Here's how the part is built. I have some questions about the finished solid (model axes, mm). A direction names the side the tool comes from. Round coordinates to 2 decimals unless told otherwise and drop trailing zeros. Loops run counter-clockwise (first coordinate to the right, second up) from the corner with the lowest first, then second, coordinate; pieces in that order, holes last. Notation, with made-up numbers: M -28.75,-11.5 L 30.25,-11.5 A15 cw 30.25,5.5 Z; hole C 72.25,42.25 d1. An arc over 180 degrees is marked long. Write each question's results on one line, items separated by ' | '. Start each with the question number.
```python
from build123d import *

# Parameters (mm, degrees)
F0_W     = 19.05
F0_H     = 6.901241
F1_DEPTH = 6.35


with BuildPart() as f1:
    # F0 (on Front) → F1 (new body)
    with BuildSketch(Plane.XZ):
        Polygon((-82.641583, -23.385886), (-82.641583, -105.935886), (-146.141583, -169.435886), (-266.791583, -169.435886), (-266.791583, -175.785886), (-273.141583, -175.785886), (-273.141583, -169.435886), (-292.191583, -169.435886), (-292.191583, -175.785886), (-298.541583, -175.785886), (-298.541583, -123.398386), (-303.509617, -123.398386), (-317.591583, -135.214559), (-331.673549, -123.398386), (-336.641583, -123.398386), (-336.641583, -207.535886), (-320.766583, -207.535886), (-320.766583, -194.835886), (-314.416583, -194.835886), (-314.416583, -207.535886), (-295.366583, -207.535886), (-184.241583, -207.535886), (-165.191583, -207.535886), (-44.541583, -207.535886), (-25.491583, -207.535886), (-6.441583, -207.535886), (-6.441583, -169.435886), (-12.791583, -169.435886), (-12.791583, -175.785886), (-19.141583, -175.785886), (-19.141583, -169.435886), (-38.191583, -169.435886), (-38.191583, -175.785886), (-44.541583, -175.785886), (-44.541583, 2.014114), (-50.891583, 2.014114), (-50.891583, 8.364114), (-44.541583, 8.364114), (-44.541583, 27.414114), (-50.891583, 27.414114), (-50.891583, 33.764114), (-44.541583, 33.764114), (-44.541583, 46.464114), (-170.452095, 46.464114), (-182.887741, 34.028468), (-169.417357, 20.558084), (-213.361327, -23.385886), align=None)
        with Locations((-304.891583, -210.986506)):
            Rectangle(F0_W, F0_H)
        with Locations((-174.716583, -210.986506)):
            Rectangle(F0_W, F0_H)
        with Locations((-35.016583, -210.986506)):
            Rectangle(F0_W, F0_H)
    extrude(amount=F1_DEPTH)


solid = f1.part
```
1. I need wall thicknesses on line 1 along Z through (x, y) = (-47, -0.25); line 2 along X through (y, z) = (-5.5, -133); line 3 along Z through (x, y) = (-294, -6). Which ranges of each line are inside material? Lowest first, please.
2. I want a section at B-B on z = -152.5. List the corners of the cut face in (x, y) for me, plus the area to 3 significant figures.
3. If we mould it in two halves opening along X, with no side actions, what happens to faces 1 (the face through (-106, -3, -207.536)), 2 (the face through (-25.492, -3, -211)), 3 (the face through (-336.642, -3, -165))? For each: released by +X, released by -X, zero draft, split by the parting line, or undercut.
4. I want a section at D-D on z = -54. List the corners of the cut face in (x, y) for me.
5. Which directions (+Z, -Z, +X, -X, +Y, -Y) give clear straight access to the entire face, cutting with the end or side of a thin tool? Please do faces 4 (the face through (-29, -3, -169.436)), 5 (the face through (-329, -3, -207.536)), 6 (the face through (-38.192, -3, -173)), 7 (the face through (-314.417, -3, -204)).
6. I want a section at C-C on x = -286. List the corners of the cut face in (y, z) for me.
7. I want a section at A-A on x = -137.5. List the corners of the cut face in (y, z) for me, plus the area to 3 significant figures.
8. For pin 1 (1 mm diameter, centred on y = -2, z = -31.5, fed in from +X); pin 2 (3 mm diameter, centred on x = -266.5, y = -4.5, fed in from -Z); pin 3 (1.9 mm diameter, centred on y = -1.5, z = -210, fed in from +X); pin 4 (2 mm diameter, centred on x = -47.5, z = -12.5, fed in from +Y), each with a flat end and sliding along its axis, tell me the tip position at first contact or that it passes through.
Outcome:
1) line 1: -207.54 to 2.01, 8.36 to 27.41, 33.76 to 46.46 | line 2: -336.64 to -320.23, -314.95 to -298.54, -109.71 to -44.54 | line 3: -207.54 to -175.79
2) outline: M -336.64,-6.35 L -298.54,-6.35 L -298.54,0 L -336.64,0 Z; M -129.21,-6.35 L -44.54,-6.35 L -44.54,0 L -129.21,0 Z | area: 780 mm2
3) face 1: undercut | face 2: released by +X | face 3: released by -X
4) outline: M -82.64,-6.35 L -44.54,-6.35 L -44.54,0 L -82.64,0 Z
5) face 4: +Z, +X, +Y, -Y | face 5: -Z, -X, +Y, -Y | face 6: +Z, +Y, -Y | face 7: -Z, +Y, -Y
6) outline: M -6.35,-207.54 L 0,-207.54 L 0,-169.44 L -6.35,-169.44 Z
7) outline: M -6.35,-207.54 L 0,-207.54 L 0,-160.79 L -6.35,-160.79 Z; M -6.35,-23.39 L 0,-23.39 L 0,46.46 L -6.35,46.46 Z | area: 740 mm2
8) pin 1: x = -44.54 | pin 2: z = -207.54 | pin 3: x = -25.49 | pin 4: y = 0
